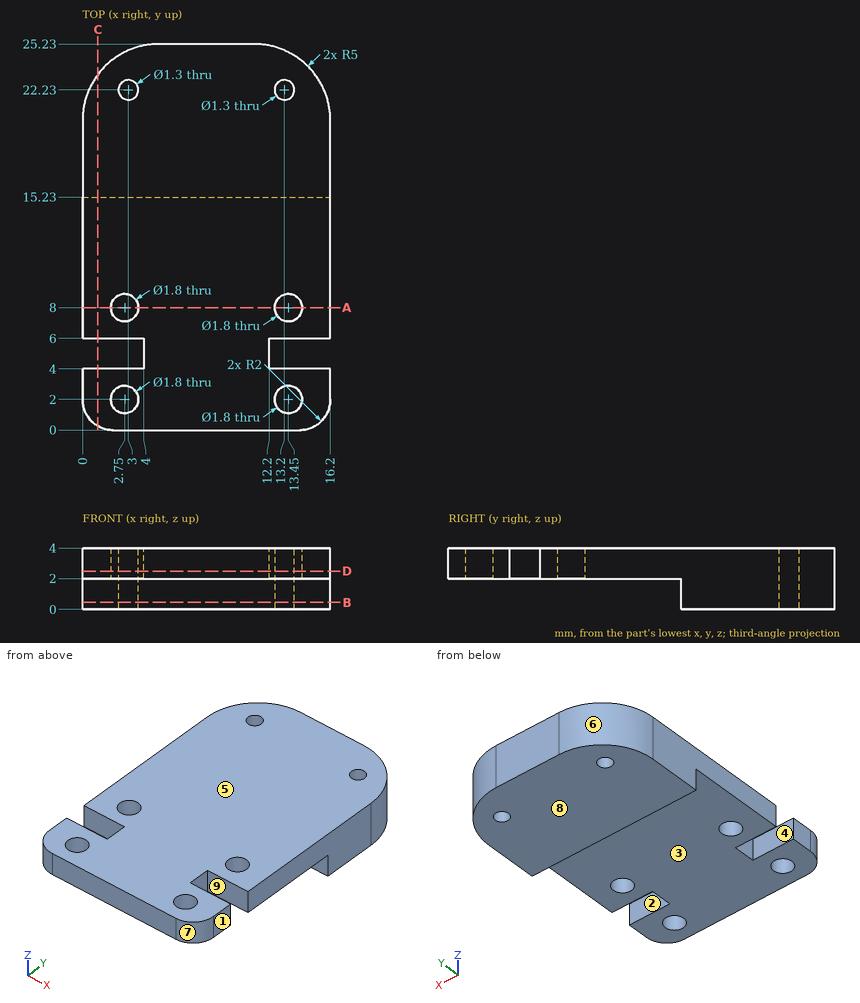
Source: three-view drawing plus pictorial views. Frame: mm from the lowest corner of the part. A direction names the side the tool comes from. Coordinates: 2 decimals unless noted, no trailing zeros. Loops run counter-clockwise (first coordinate to the right, second up) from the corner with the lowest first, then second, coordinate; pieces in that order, holes last. Notation, with made-up numbers: (-13.5, 41.5) - (-7.5, 41.5) arc R24 ccw to (-7.5, 68.5) - close; hole circle Ø4 at (57.25, 47). An arc over 180 degrees is marked (long way). Answer in a Markdown table with one row per item. Add a question column.
Item 1: Contact query for flat-ended pins moving along their axis: P1, Ø0.6, axis at x = 1.5, z = 3, coming from the -Y side; P2, Ø1, axis at x = 7, z = 1, coming from the -Y side; P3, Ø1, axis at x = 1.5, z = 3, coming from the +Y side; P4, Ø1.4, axis at x = 13.45, y = 8, coming from the -Z side. Output: stop coordinate, or through.
Item 2: Section query A-A on y = 8. Return the cut outline in (x, z).
Item 3: Access query for the marked faces 1, 2, 3, 4 and 5. Directions: +Z, -Z, +X, -X, +Y, -Y. A direction counts if a zero-diameter tool reaches every point of the face in a straight line with its end or side. Return the directions, or none.
Item 4: Mould query, pull axis Y, two halves, no side actions, for the marked faces 6, 7, 8 and 9. Classes: released by +Y, released by -Y, zero draft, split by the parting line, or undercut.
Item 5: Section query B-B on z = 0.45. Return the cut outline in (x, y), then the cut area to 3 significant figures.
Item 6: Section query C-C on x = 1. Return the cut outline in (y, z), then the cut area to 3 significant figures.
Item 7: Section query D-D on z = 2.5. Return the cut outline in (x, y).
Item 8: Line query: line 1 along X through (y, z) = (2, 3.2); line 2 along Y through (x, z) = (13.2, 2.15); line 3 along Y through (x, z) = (12.75, 2.95). Output: solid intervals per line, ascending. Write a range as [from, to].
Recorded:
| question | item | result |
|---|---|---|
| 1 | P1 | y = 0.01 |
| 1 | P2 | y = 15.23 |
| 1 | P3 | y = 24.23 |
| 1 | P4 | through |
| 2 | outline | (0, 2) - (1.85, 2) - (1.85, 4) - (0, 4) - close; (3.65, 2) - (12.55, 2) - (12.55, 4) - (3.65, 4) - close; (14.35, 2) - (16.2, 2) - (16.2, 4) - (14.35, 4) - close |
| 3 | face 1 | +Z, -Z, +X, +Y, -Y |
| 3 | face 2 | +Z, -Z, +X |
| 3 | face 3 | -Z, +X, -X, -Y |
| 3 | face 4 | +Z, -Z, -X |
| 3 | face 5 | +Z, +X, -X, +Y, -Y |
| 4 | face 6 | released by +Y |
| 4 | face 7 | released by -Y |
| 4 | face 8 | zero draft |
| 4 | face 9 | undercut |
| 5 | outline | (0, 15.23) - (16.2, 15.23) - (16.2, 20.23) arc R5 ccw to (11.2, 25.23) - (5, 25.23) arc R5 ccw to (0, 20.23) - close; hole circle Ø1.3 at (3, 22.23); hole circle Ø1.3 at (13.2, 22.23) |
| 5 | area | 149 mm^2 |
| 6 | outline | (0.27, 2) - (4, 2) - (4, 4) - (0.27, 4) - close; (6, 2) - (15.23, 2) - (15.23, 0) - (23.23, 0) - (23.23, 4) - (6, 4) - close |
| 6 | area | 57.9 mm^2 |
| 7 | outline | (0, 2) arc R2 ccw to (2, 0) - (14.2, 0) arc R2 ccw to (16.2, 2) - (16.2, 4) - (12.2, 4) - (12.2, 6) - (16.2, 6) - (16.2, 20.23) arc R5 ccw to (11.2, 25.23) - (5, 25.23) arc R5 ccw to (0, 20.23) - (0, 6) - (4, 6) - (4, 4) - (0, 4) - close; hole circle Ø1.8 at (2.75, 2); hole circle Ø1.8 at (2.75, 8); hole circle Ø1.3 at (3, 22.23); hole circle Ø1.8 at (13.45, 2); hole circle Ø1.8 at (13.45, 8); hole circle Ø1.3 at (13.2, 22.23) |
| 8 | line 1 | [0, 1.85], [3.65, 12.55], [14.35, 16.2] |
| 8 | line 2 | [0, 1.14], [2.86, 4], [6, 7.14], [8.86, 21.58], [22.88, 24.81] |
| 8 | line 3 | [0, 1.43], [2.57, 4], [6, 7.43], [8.57, 21.76], [22.7, 24.98] |
